```python
from build123d import *

# Parameters (mm, degrees)
F0_R     = 9.33
F1_DEPTH = 15
F2_DEPTH = 10


with BuildPart() as f1:
    # F0 (on Front) → F1 (new body)
    with BuildSketch(Plane.XZ):
        with BuildLine():
            ThreePointArc((-12.417365469, 39.4797180027), (-10.928240176, 42.6488659683), (-10.417365469, 46.1129675834))
            ThreePointArc((-10.417365469, 46.1129675834), (-22.417365469, 58.1129675834), (-34.417365469, 46.1129675834))
            ThreePointArc((-34.417365469, 46.1129675834), (-33.9064907621, 42.6488659683), (-32.417365469, 39.4797180027))
            ThreePointArc((-32.417365469, 39.4797180027), (-22.417365469, 34.1129675834), (-12.417365469, 39.4797180027))
        make_face()
        with Locations((-22.417365469, 46.1129675834)):
            Circle(F0_R, mode=Mode.SUBTRACT)
        with BuildLine():
            Line((-10.417365469, 0), (-10.417365469, 46.1129675834))
            ThreePointArc((-10.417365469, 46.1129675834), (-10.928240176, 42.6488659683), (-12.417365469, 39.4797180027))
            Line((-12.417365469, 39.4797180027), (-12.417365469, 2))
            Line((-12.417365469, 2), (-32.417365469, 2))
            Line((-32.417365469, 2), (-32.417365469, 39.4797180027))
            ThreePointArc((-32.417365469, 39.4797180027), (-33.9064907621, 42.6488659683), (-34.417365469, 46.1129675834))
            Line((-34.417365469, 46.1129675834), (-34.417365469, 0))
            Line((-34.417365469, 0), (-10.417365469, 0))
        make_face()
    extrude(amount=F1_DEPTH)

    # F0 (on Front) → F2 (join)
    with BuildSketch(Plane.XZ):
        with BuildLine():
            Line((-12.417365469, 2), (-12.417365469, 39.4797180027))
            ThreePointArc((-12.417365469, 39.4797180027), (-22.417365469, 34.1129675834), (-32.417365469, 39.4797180027))
            Line((-32.417365469, 39.4797180027), (-32.417365469, 2))
            Line((-32.417365469, 2), (-12.417365469, 2))
        make_face()
        with BuildLine():
            add(Edge.make_bspline(
                [(-22.9718386234, 19.2682127741), (-23.2651889221, 19.2059506699), (-23.6806687329, 19.2059506699)],
                knots=[0, 0, 0, 1, 1, 1], degree=2))
            add(Edge.make_bspline(
                [(-23.6806687329, 19.2059506699), (-24.5894559848, 19.2059506699), (-25.1156905003, 19.760322867)],
                knots=[0, 0, 0, 1, 1, 1], degree=2))
            add(Edge.make_bspline(
                [(-25.1156905003, 19.760322867), (-25.6419250157, 20.3146950642), (-25.6419250157, 21.2977179019)],
                knots=[0, 0, 0, 1, 1, 1], degree=2))
            add(Edge.make_bspline(
                [(-25.6419250157, 21.2977179019), (-25.6419250157, 22.2903195249), (-25.1534069672, 22.8740267519)],
                knots=[0, 0, 0, 1, 1, 1], degree=2))
            add(Edge.make_bspline(
                [(-25.1534069672, 22.8740267519), (-24.6648889188, 23.4577339789), (-23.8411133861, 23.4577339789)],
                knots=[0, 0, 0, 1, 1, 1], degree=2))
            add(Edge.make_bspline(
                [(-23.8411133861, 23.4577339789), (-23.0712185205, 23.4577339789), (-22.6222129612, 22.950657034)],
                knots=[0, 0, 0, 1, 1, 1], degree=2))
            add(Edge.make_bspline(
                [(-22.6222129612, 22.950657034), (-22.173207402, 22.4435800891), (-22.173207402, 21.6126204674)],
                knots=[0, 0, 0, 1, 1, 1], degree=2))
            Line((-22.173207402, 21.6126204674), (-22.173207402, 21.2198902716))
            Line((-22.173207402, 21.2198902716), (-24.9977517067, 21.2198902716))
            add(Edge.make_bspline(
                [(-24.9977517067, 21.2198902716), (-24.9785941362, 20.4978893323), (-24.6325605185, 20.123718033)],
                knots=[0, 0, 0, 1, 1, 1], degree=2))
            add(Edge.make_bspline(
                [(-24.6325605185, 20.123718033), (-24.2865269008, 19.7495467336), (-23.6579191179, 19.7495467336)],
                knots=[0, 0, 0, 1, 1, 1], degree=2))
            add(Edge.make_bspline(
                [(-23.6579191179, 19.7495467336), (-22.9957855865, 19.7495467336), (-22.3492175812, 20.0261341581)],
                knots=[0, 0, 0, 1, 1, 1], degree=2))
            Line((-22.3492175812, 20.0261341581), (-22.3492175812, 19.4717619609))
            add(Edge.make_bspline(
                [(-22.3492175812, 19.4717619609), (-22.6784883246, 19.3304748783), (-22.9718386234, 19.2682127741)],
                knots=[0, 0, 0, 1, 1, 1], degree=2))
        make_face(mode=Mode.SUBTRACT)
        Polygon((-28.3539185936, 22.3753312441), (-26.0717730044, 19.2813836038), (-26.8201156032, 19.2813836038), (-28.8137002863, 21.9347071219), (-29.3872300539, 21.4258341548), (-29.3872300539, 19.2813836038), (-30.0230219258, 19.2813836038), (-30.0230219258, 24.7520673377), (-29.3872300539, 24.7520673377), (-29.3872300539, 22.0388764117), (-26.9063246706, 24.7520673377), (-26.1543900273, 24.7520673377), align=None, mode=Mode.SUBTRACT)
        with BuildLine():
            Line((-20.1101765257, 19.2586339888), (-21.7649116801, 23.382301045))
            Line((-21.7649116801, 23.382301045), (-21.0979887561, 23.382301045))
            Line((-21.0979887561, 23.382301045), (-20.1999776376, 21.0438800924))
            add(Edge.make_bspline(
                [(-20.1999776376, 21.0438800924), (-19.9054299907, 20.2428541747), (-19.8335891012, 19.8872417718)],
                knots=[0, 0, 0, 1, 1, 1], degree=2))
            Line((-19.8335891012, 19.8872417718), (-19.8036553973, 19.8872417718))
            add(Edge.make_bspline(
                [(-19.8036553973, 19.8872417718), (-19.755761471, 20.078817477), (-19.6001062104, 20.540993866)],
                knots=[0, 0, 0, 1, 1, 1], degree=2))
            add(Edge.make_bspline(
                [(-19.6001062104, 20.540993866), (-19.4444509499, 21.003170255), (-18.5835576243, 23.382301045)],
                knots=[0, 0, 0, 1, 1, 1], degree=2))
            Line((-18.5835576243, 23.382301045), (-17.9178320484, 23.382301045))
            Line((-17.9178320484, 23.382301045), (-19.680328537, 18.7126432288))
            add(Edge.make_bspline(
                [(-19.680328537, 18.7126432288), (-19.9425477836, 18.0205759934), (-20.2921734457, 17.7302190651)],
                knots=[0, 0, 0, 1, 1, 1], degree=2))
            add(Edge.make_bspline(
                [(-20.2921734457, 17.7302190651), (-20.6417991079, 17.4398621368), (-21.150672075, 17.4398621368)],
                knots=[0, 0, 0, 1, 1, 1], degree=2))
            add(Edge.make_bspline(
                [(-21.150672075, 17.4398621368), (-21.4356409366, 17.4398621368), (-21.7122283611, 17.5045189373)],
                knots=[0, 0, 0, 1, 1, 1], degree=2))
            Line((-21.7122283611, 17.5045189373), (-21.7122283611, 18.0014184229))
            add(Edge.make_bspline(
                [(-21.7122283611, 18.0014184229), (-21.506284478, 17.9571165411), (-21.2524466685, 17.9571165411)],
                knots=[0, 0, 0, 1, 1, 1], degree=2))
            add(Edge.make_bspline(
                [(-21.2524466685, 17.9571165411), (-20.6118654039, 17.9571165411), (-20.3388700239, 18.6755254359)],
                knots=[0, 0, 0, 1, 1, 1], degree=2))
            Line((-20.3388700239, 18.6755254359), (-20.1101765257, 19.2586339888))
        make_face(mode=Mode.SUBTRACT)
        with BuildLine():
            add(Edge.make_bspline(
                [(-14.8633968974, 21.0774058408), (-14.6071643915, 20.8080025053), (-14.6071643915, 20.3997067834)],
                knots=[0, 0, 0, 1, 1, 1], degree=2))
            add(Edge.make_bspline(
                [(-14.6071643915, 20.3997067834), (-14.6071643915, 19.8273743639), (-15.0334203358, 19.5166625169)],
                knots=[0, 0, 0, 1, 1, 1], degree=2))
            add(Edge.make_bspline(
                [(-15.0334203358, 19.5166625169), (-15.45967628, 19.2059506699), (-16.2307684938, 19.2059506699)],
                knots=[0, 0, 0, 1, 1, 1], degree=2))
            add(Edge.make_bspline(
                [(-16.2307684938, 19.2059506699), (-17.0461625894, 19.2059506699), (-17.5023522376, 19.464577872)],
                knots=[0, 0, 0, 1, 1, 1], degree=2))
            Line((-17.5023522376, 19.464577872), (-17.5023522376, 20.040502336))
            add(Edge.make_bspline(
                [(-17.5023522376, 20.040502336), (-17.2066072426, 19.8908338162), (-16.8683563879, 19.8052234229)],
                knots=[0, 0, 0, 1, 1, 1], degree=2))
            add(Edge.make_bspline(
                [(-16.8683563879, 19.8052234229), (-16.5301055333, 19.7196130296), (-16.2152029677, 19.7196130296)],
                knots=[0, 0, 0, 1, 1, 1], degree=2))
            add(Edge.make_bspline(
                [(-16.2152029677, 19.7196130296), (-15.7290796156, 19.7196130296), (-15.4674590431, 19.8746696161)],
                knots=[0, 0, 0, 1, 1, 1], degree=2))
            add(Edge.make_bspline(
                [(-15.4674590431, 19.8746696161), (-15.2058384705, 20.0297262026), (-15.2058384705, 20.3482208126)],
                knots=[0, 0, 0, 1, 1, 1], degree=2))
            add(Edge.make_bspline(
                [(-15.2058384705, 20.3482208126), (-15.2058384705, 20.5876904442), (-15.4129797019, 20.7577138826)],
                knots=[0, 0, 0, 1, 1, 1], degree=2))
            add(Edge.make_bspline(
                [(-15.4129797019, 20.7577138826), (-15.6201209332, 20.9277373211), (-16.2235844048, 21.1600228637)],
                knots=[0, 0, 0, 1, 1, 1], degree=2))
            add(Edge.make_bspline(
                [(-16.2235844048, 21.1600228637), (-16.7959168244, 21.3731508358), (-17.0371824782, 21.5323981409)],
                knots=[0, 0, 0, 1, 1, 1], degree=2))
            add(Edge.make_bspline(
                [(-17.0371824782, 21.5323981409), (-17.278448132, 21.6916454459), (-17.3963869256, 21.8933986105)],
                knots=[0, 0, 0, 1, 1, 1], degree=2))
            add(Edge.make_bspline(
                [(-17.3963869256, 21.8933986105), (-17.5143257192, 22.0951517751), (-17.5143257192, 22.3753312441)],
                knots=[0, 0, 0, 1, 1, 1], degree=2))
            add(Edge.make_bspline(
                [(-17.5143257192, 22.3753312441), (-17.5143257192, 22.8770201223), (-17.1060299973, 23.1673770506)],
                knots=[0, 0, 0, 1, 1, 1], degree=2))
            add(Edge.make_bspline(
                [(-17.1060299973, 23.1673770506), (-16.6977342754, 23.4577339789), (-15.9877068177, 23.4577339789)],
                knots=[0, 0, 0, 1, 1, 1], degree=2))
            add(Edge.make_bspline(
                [(-15.9877068177, 23.4577339789), (-15.3255732863, 23.4577339789), (-14.6921761108, 23.1883306434)],
                knots=[0, 0, 0, 1, 1, 1], degree=2))
            Line((-14.6921761108, 23.1883306434), (-14.91368552, 22.6830497207))
            add(Edge.make_bspline(
                [(-14.91368552, 22.6830497207), (-15.5303198214, 22.9368875302), (-16.0320086996, 22.9368875302)],
                knots=[0, 0, 0, 1, 1, 1], degree=2))
            add(Edge.make_bspline(
                [(-16.0320086996, 22.9368875302), (-16.4738301699, 22.9368875302), (-16.6983329495, 22.7985938179)],
                knots=[0, 0, 0, 1, 1, 1], degree=2))
            add(Edge.make_bspline(
                [(-16.6983329495, 22.7985938179), (-16.9228357291, 22.6603001057), (-16.9228357291, 22.4172384296)],
                knots=[0, 0, 0, 1, 1, 1], degree=2))
            add(Edge.make_bspline(
                [(-16.9228357291, 22.4172384296), (-16.9228357291, 22.2520043838), (-16.838422684, 22.1364602866)],
                knots=[0, 0, 0, 1, 1, 1], degree=2))
            add(Edge.make_bspline(
                [(-16.838422684, 22.1364602866), (-16.7540096388, 22.0209161893), (-16.5672233262, 21.9161482255)],
                knots=[0, 0, 0, 1, 1, 1], degree=2))
            add(Edge.make_bspline(
                [(-16.5672233262, 21.9161482255), (-16.3804370135, 21.8113802617), (-15.8488144314, 21.6126204674)],
                knots=[0, 0, 0, 1, 1, 1], degree=2))
            add(Edge.make_bspline(
                [(-15.8488144314, 21.6126204674), (-15.1196294032, 21.3468091764), (-14.8633968974, 21.0774058408)],
                knots=[0, 0, 0, 1, 1, 1], degree=2))
        make_face(mode=Mode.SUBTRACT)
    extrude(amount=F2_DEPTH)


solid = f1.part
```
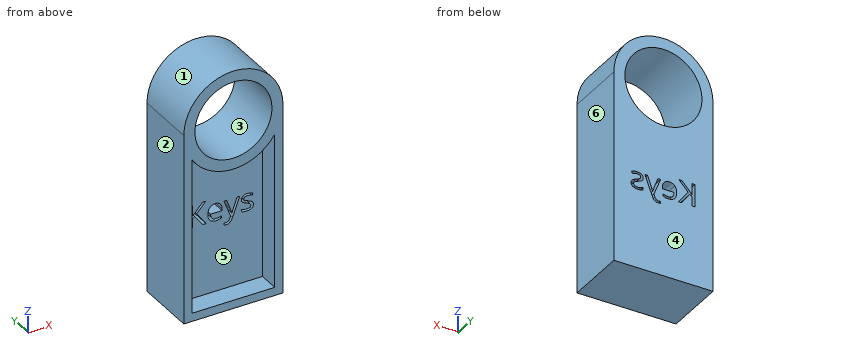
Input: part model. Units: mm. Frame: model coordinates. Face numbers are marked on the shaded views. A direction names the side the tool comes from. Give positions to 0.01 mm unless a question says otherwise; leave off trailing zeros. Loops run counter-clockwise (first coordinate to the right, second up) from the corner with the lowest first, then second, coordinate; pieces in that order, holes last.
1) Section query B-B on z = 47. Return the cut outline in (x, y).
A:
outline: (-34.38, -15) - (-31.71, -15) - (-31.71, 0) - (-34.38, 0) - close; (-13.13, -15) - (-10.45, -15) - (-10.45, 0) - (-13.13, 0) - close
2) Section query C-C on z = 11. Return the cut outline in (x, y).
A:
outline: (-34.42, -15) - (-32.42, -15) - (-32.42, -10) - (-12.42, -10) - (-12.42, -15) - (-10.42, -15) - (-10.42, 0) - (-34.42, 0) - close
3) Section query A-A on y = -14. Return the cut outline in (x, z), and give its area (3 significant figures).
A:
outline: (-34.42, 0) - (-10.42, 0) - (-10.42, 46.11) arc R12 ccw to (-34.42, 46.11) - close; hole (-32.42, 2) - (-12.42, 2) - (-12.42, 39.48) arc R12 cw to (-32.42, 39.48) - close; hole circle Ø18.66 at (-22.42, 46.11)
area: 385 mm2
4) Contact query for flat-ended pins moving along their axis: pin 1 (1.5 mm diameter, centred on x = -21.5, z = 6, fed in from -Y); pin 2 (2 mm diameter, centred on x = -21, y = -12.5, fed in from +Z). Output: stop coordinate, or through.
A:
pin 1: stops at y = -10
pin 2: stops at z = 58.11
5) Mould query, pull axis X, two halves, no side actions, for the marked faces 1, 2, 3 and 4. Classes: released by +X, released by -X, zero draft, split by the parting line, or undercut.
A:
face 1: split by the parting line
face 2: released by -X
face 3: undercut
face 4: zero draft
6) Reachability of the marked faces 5 and 6 from +Z, -Z, +X, -X, +Y, -Y: full face, straight path, thin tool, end or side. Return the list, or none.
A:
face 5: -Y
face 6: +Z, -Z, +X, +Y, -Y
7) Section query D-D on x = -24. Count the separate pieces of the cut face and the enclosed holes in it, and give its area (3 significant figures).
A:
separate pieces: 4
enclosed holes: 0
area: 405 mm2
8) Line query: L1, parallel to X at y = -11.5, z = 13; L2, parallel to Z at x = -26.75, y = -7.5; L3, parallel to Z at x = -28.5, y = -9.75. Output: solid intervals per line, ascending.
A:
L1: x = -34.42 to -32.42, -12.42 to -10.42
L2: z = 0 to 19.28, 20.2 to 24.11, 24.75 to 37.85, 54.38 to 57.3
L3: z = 0 to 21.52, 23.01 to 39.04, 53.19 to 56.46
